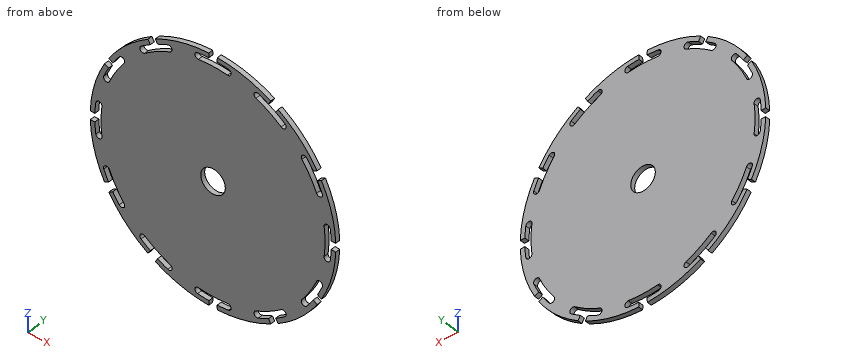
```python
from build123d import *

# Parameters (mm, degrees)
SKETCH1_R         = 40
WHEEL_BLANK_DEPTH = 1.5
T_SLOT_DEPTH      = 2.5
CIRPATTERN_COUNT  = 12
SKETCH3_R         = 4
CENTER_HOLE_DEPTH = 6


with BuildPart() as part:
    # Sketch1 → Wheel Blank (new body)
    with BuildSketch(Plane(origin=(0, 0, 0), x_dir=(1, 0, 0), z_dir=(0, 1, 0))):
        Circle(SKETCH1_R)
    extrude(amount=WHEEL_BLANK_DEPTH)

    # Sketch2 → T-Slot (cut, through all)
    with BuildSketch(Plane(origin=(0, 0, 0), x_dir=(1, 0, 0), z_dir=(0, 1, 0))):
        with BuildLine():
            Line((-1.395979868, 39.975633081), (-1.343630623, 38.47654684))
            ThreePointArc((-1.343630623, 38.47654684), (-3.188115989, 38.367771846), (-5.0252584, 38.170627163))
            ThreePointArc((-5.0252584, 38.170627163), (-5.88617707, 37.048656109), (-4.764206016, 36.18773744))
            ThreePointArc((-4.764206016, 36.18773744), (0, 36.5), (4.764206016, 36.18773744))
            ThreePointArc((4.764206016, 36.18773744), (5.88617707, 37.048656109), (5.0252584, 38.170627163))
            ThreePointArc((5.0252584, 38.170627163), (3.188115989, 38.367771846), (1.343630623, 38.47654684))
            Line((1.343630623, 38.47654684), (1.395979868, 39.975633081))
            ThreePointArc((1.395979868, 39.975633081), (0, 40), (-1.395979868, 39.975633081))
        make_face()
    t_slot = extrude(amount=T_SLOT_DEPTH, mode=Mode.SUBTRACT)

    # CirPattern: T-Slot ×12 about axis
    cirpattern_axis = Axis((0, 0, 0), (0, 1, 0))
    for i in range(1, CIRPATTERN_COUNT):
        add(t_slot.rotate(cirpattern_axis, i * 360 / CIRPATTERN_COUNT), mode=Mode.SUBTRACT)

    # Sketch3 → Center Hole (cut)
    with BuildSketch(Plane(origin=(0, 0, 0), x_dir=(1, 0, 0), z_dir=(0, 1, 0))):
        Circle(SKETCH3_R)
    extrude(amount=CENTER_HOLE_DEPTH, mode=Mode.SUBTRACT)


solid = part.part
```
The model under review builds one solid part; all positions refer to its coordinate system, in mm. Coordinates: 2 decimals unless noted, no trailing zeros. Write each loop counter-clockwise with the first axis right and the second up, starting at its lowest first coordinate (ties: lowest second). Pieces come first, ordered by that corner, then holes. Notation, with made-up numbers: (-4, 17.5) - (40, 17.5) arc R8 ccw to (40, 32.5) - close; hole circle Ø6 at (-19.75, 7). An arc over 180 degrees is marked (long way). Answer in a Markdown table with one row per item. Add a question column.
Q1. To check wall thickness, follow line 1 along Z through (x, y) = (0, 0.55); line 2 along Z through (x, y) = (21, 1.3). State the ranges of each line that lie inside material, in increasing order. Write a range as from..to.
Q2. Consider section A-A on x = 0. Give the boundary of the cut face in (y, z), then the cut area to 3 significant figures.
Q3. Consider section C-C on z = 16. Give the boundary of the cut face in (x, y), then the cut area to 3 significant figures.
Q4. Consider section B-B on z = 0. Give the boundary of the cut face in (x, y).
Q5. Consider section D-D on x = -11.5. Give the boundary of the cut face in (y, z).
Q6. Clearance check with flat-ended pins moving along their axes: pin 1 (5 mm diameter, centred on x = 0, z = 0, fed in from +Y); pin 2 (8 mm diameter, centred on x = 12, z = 15.5, fed in from -Y). State where each tip first meets the part, or that it passes through.
Answers below:
| question | item | result |
|---|---|---|
| 1 | line 1 | -36.5..-4, 4..36.5 |
| 1 | line 2 | -33.61..-32.27, -29.85..29.85, 32.27..33.61 |
| 2 | outline | (0, -36.5) - (1.5, -36.5) - (1.5, -4) - (0, -4) - close; (0, 4) - (1.5, 4) - (1.5, 36.5) - (0, 36.5) - close |
| 2 | area | 97.5 mm² |
| 3 | outline | (-36.66, 0) - (-35.02, 0) - (-35.02, 1.5) - (-36.66, 1.5) - close; (-32.81, 0) - (32.81, 0) - (32.81, 1.5) - (-32.81, 1.5) - close; (35.02, 0) - (36.66, 0) - (36.66, 1.5) - (35.02, 1.5) - close |
| 3 | area | 103 mm² |
| 4 | outline | (-36.5, 0) - (-4, 0) - (-4, 1.5) - (-36.5, 1.5) - close; (4, 0) - (36.5, 0) - (36.5, 1.5) - (4, 1.5) - close |
| 5 | outline | (0, -38.31) - (1.5, -38.31) - (1.5, 38.31) - (0, 38.31) - close |
| 6 | pin 1 | through |
| 6 | pin 2 | y = 0 |
